Read the model definition and answer for the solid it produces. Units are mm, in the model's axes. Face numbers are marked on the shaded views. A direction names the side the tool comes from. Coordinates: 2 decimals unless noted, no trailing zeros. Loops run counter-clockwise (first coordinate to the right, second up) from the corner with the lowest first, then second, coordinate; pieces in that order, holes last. Notation, with made-up numbers: M 15,40 L 32,40 A24 ccw 32,73 Z; hole C 89.5,17 d8. An arc over 180 degrees is marked long. Use one line per item in the form item = value. Start each with the question number.
1. The part is cut by section A-A (y = -31). Give the vertices of the cut face in (x, z), plus the area to 3 significant figures.
2. Find the intervals of material crossed by probe 1 along Z at (x, y) = (11.4, -4); probe 2 along Y at (x, z) = (-9, 43.85); probe 3 along Z at (x, y) = (1, -13.5), in increasing order. Write a range as [from, to].
3. The part is cut by section B-B (z = 6). Give the vertices of the cut face in (x, y).
4. Flat-ended cylindrical pins translate along their axes: pin 1 (5 mm diameter, centred on x = -0.5, z = 27, fed in from -Y); pin 2 (12 mm diameter, centred on x = -7.5, z = 31.5, fed in from +Y); pin 3 (0.6 mm diameter, centred on y = -20.5, z = 44.5, fed in from -X). Find the tip coordinate at first contact, or state that the pin passes through.
5. For a pull along Z with two mould halves and no side action, classify the marked faces 1, 2, 3 and 4 as released by +Z, released by -Z, zero draft, split by the parting line, or undercut.
6. The part is cut by section D-D (y = -47). Give the vertices of the cut face in (x, z), plus the area to 3 significant figures.
7. A tool of negligible diameter and unlimited length cuts with its end or side. For the marked faces 5, 6 and 7, from which of +Z, -Z, +X, -X, +Y, -Y can it reach the whole face along a straight path? Write none if from no direction.
8. The part is cut by section C-C (x = -3). Give the vertices of the cut face in (y, z) (3 decimals).
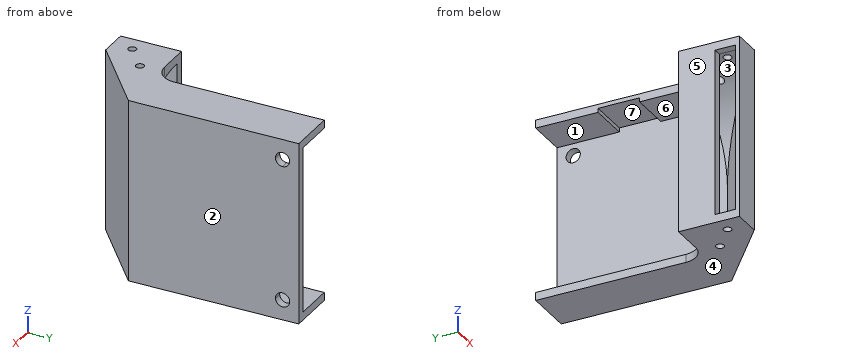
from build123d import *

# Parameters (mm, degrees)
F1_DEPTH  = 45
F3_DEPTH  = 2
F4_W      = 10
F4_H      = 42
F4_R      = 1
F5_DEPTH  = 2
F7_DEPTH  = 2
F8_R      = 5
F9_W      = 10
F9_H      = 10.2169760242
F10_DEPTH = 1
F11_W     = 9
F11_H     = 41
F12_DEPTH = 2
F16_DEPTH = 45.001


# Not quite as in the source:
# - a feature names something its author has since deleted; it is built from what else it names


with BuildPart() as f1:
    # F0 (on Top) → F1 (new body)
    with BuildSketch(Plane.XY):
        with BuildLine():
            Line((12, -42), (12, 0))
            Line((12, 0), (10, 0))
            Line((10, 0), (10, -42))
            Line((10, -42), (-4.5861525412, -54.7628834735))
            ThreePointArc((-4.5861525412, -54.7628834735), (-6.1200422145, -55.6805137201), (-7.8786755805, -56))
            Line((-7.8786755805, -56), (-13, -56))
            Line((-13, -56), (-13, -57))
            Line((-13, -57), (-6, -57))
            Line((-6, -57), (12, -42))
        make_face()
    extrude(amount=F1_DEPTH)

    # F2 (on face) → F3 (cut, through all)
    with BuildSketch(Plane(origin=(10, 0, 0), x_dir=(0, -1, 0), z_dir=(-1, 0, 0))):
        with BuildLine():
            ThreePointArc((4, 6.75), (2.7625631329, 3.7625631329), (5.75, 5))
            ThreePointArc((5.75, 5), (5.2374368671, 6.2374368671), (4, 6.75))
        make_face()
        with BuildLine():
            ThreePointArc((5.75, 40), (2.7625631329, 41.2374368671), (4, 38.25))
            ThreePointArc((4, 38.25), (5.2374368671, 38.7625631329), (5.75, 40))
        make_face()
    extrude(amount=-F3_DEPTH, mode=Mode.SUBTRACT)

    # F4 (on face) → F5 (join)
    with BuildSketch(Plane(origin=(0, 0, 0), x_dir=(1, 0, 0), z_dir=(0, 0, -1))):
        Polygon((10, 42), (12, 42), (0, 52), (0, 50.75), align=None)
        with Locations((5, 21)):
            Rectangle(F4_W, F4_H)
        Polygon((0, 42), (10, 42), (0, 50.75), align=None)
        with BuildLine():
            Line((0, 42), (0, 50.75))
            Line((0, 50.75), (-4.5861525412, 54.7628834735))
            ThreePointArc((-4.5861525412, 54.7628834735), (-6.1200422145, 55.6805137201), (-7.8786755805, 56))
            Line((-7.8786755805, 56), (-13, 56))
            Line((-13, 56), (-13, 42))
            Line((-13, 42), (0, 42))
        make_face()
        with Locations((-9, 52)):
            Circle(F4_R, mode=Mode.SUBTRACT)
        with Locations((-3, 47)):
            Circle(F4_R, mode=Mode.SUBTRACT)
        with Locations((-9, 52)):
            Circle(F4_R)
        with Locations((-3, 47)):
            Circle(F4_R)
    extrude(amount=-F5_DEPTH)

    # F6 (on face) → F7 (join)
    with BuildSketch(Plane.XY.offset(45)):
        Polygon((12, -42), (12, 0), (0, 0), (0, -42), (-13, -42), (-13, -57), (-6, -57), align=None)
    extrude(amount=-F7_DEPTH)

    # F8
    f8_edges = [f1.edges().sort_by_distance(p)[0] for p in [
        (0, -42, 44),
        (0, -42, 1),
    ]]
    fillet(f8_edges, radius=F8_R)

    # F9 (on face) → F10 (cut)
    with BuildSketch(Plane(origin=(0, 0, 43), x_dir=(1, 0, 0), z_dir=(0, 0, -1))):
        with Locations((5, 20.4747493975)):
            Rectangle(F9_W, F9_H)
    extrude(amount=-F10_DEPTH, mode=Mode.SUBTRACT)

    # F11 (on face) → F12 (join)
    with BuildSketch(Plane(origin=(-13, 0, 0), x_dir=(0, -1, 0), z_dir=(-1, 0, 0))):
        with Locations((46.5, 22.5)):
            Rectangle(F11_W, F11_H)
    extrude(amount=-F12_DEPTH)

    # F14 (on offset) → F15 (join, up to the next surface of F1)
    with BuildSketch(Plane.XZ.offset(42)):
        with BuildLine():
            ThreePointArc((-11, 43), (3.8492424049, 36.8492424049), (10, 22))
            Line((10, 22), (10, 43))
            Line((10, 43), (-11, 43))
        make_face()
    extrude(until=Until.NEXT)

    # F4 (on face) → F16 (cut, through all)
    with BuildSketch(Plane(origin=(0, 0, 0), x_dir=(1, 0, 0), z_dir=(0, 0, -1))):
        with Locations((-3, 47)):
            Circle(F4_R)
        with Locations((-9, 52)):
            Circle(F4_R)
    extrude(amount=-F16_DEPTH, mode=Mode.SUBTRACT)


solid = f1.part
Computed values:
q1.outline = M 0,0 L 12,0 L 12,45 L 0,45 L 0,43 L 10,43 L 10,2 L 0,2 Z
q1.area = 130 mm²
q2.probe_1 = [0, 3.25], [6.75, 38.25], [41.75, 45]
q2.probe_2 = [-57, -53], [-51, -42]
q2.probe_3 = [0, 2], [43, 45]
q3.outline = M -13,-57 L -6,-57 L 12,-42 L 12,-5.44 L 10,-5.44 L 10,-42 L -4.59,-54.76 A5 cw -7.88,-56 L -13,-56 Z; M -13,-51 L -11,-51 L -11,-42 L -13,-42 Z; M 10,-2.56 L 12,-2.56 L 12,0 L 10,0 Z
q4.pin_1 = -54.5
q4.pin_2 = -42
q4.pin_3 = 0
q5.face_1 = undercut
q5.face_2 = zero draft
q5.face_3 = undercut
q5.face_4 = released by -Z
q6.outline = M -13,0 L -4,0 L -4,2 L -11,2 L -11,43 A21 cw -4,41.8 L -4,45 L -13,45 Z; M -2,0 L 6,0 L 6,45 L -2,45 L -2,40.97 A21 cw 4.29,36.4 L 4.29,2 L -2,2 Z
q6.area = 248 mm²
q7.face_5 = +Z, -Z, -X, +Y, -Y
q7.face_6 = -X, +Y
q7.face_7 = -X
q8.outline = M -54.5,0 L -48,0 L -48,2 L -53.375,2 L -53.375,41.416 L -48,41.416 L -48,45 L -54.5,45 Z; M -46,0 L -41.583,0 L -41.583,2 L -46,2 Z; M -46,41.416 L -42,41.416 L -42,43 L -41.583,43 L -41.583,45 L -46,45 Z
